Geometry: see drawing. Coordinates: mm, zero at the bounding-box minimum. A direction names the side the tool comes from. Give positions to 0.01 mm unless a question says otherwise; leave off trailing zeros. Order: outer loops, then holes, each group sorted by start corner. A loop starts at its lowest first (then second) coordinate and runs counter-clockwise, first axis right, second up. Notation, with made-up numbers: (26, 70) - (66, 70) arc R15 cw to (66, 75) - close; hole circle Ø9 at (72.25, 59). An arc over 180 degrees is marked (long way). One line per item, written item: value.
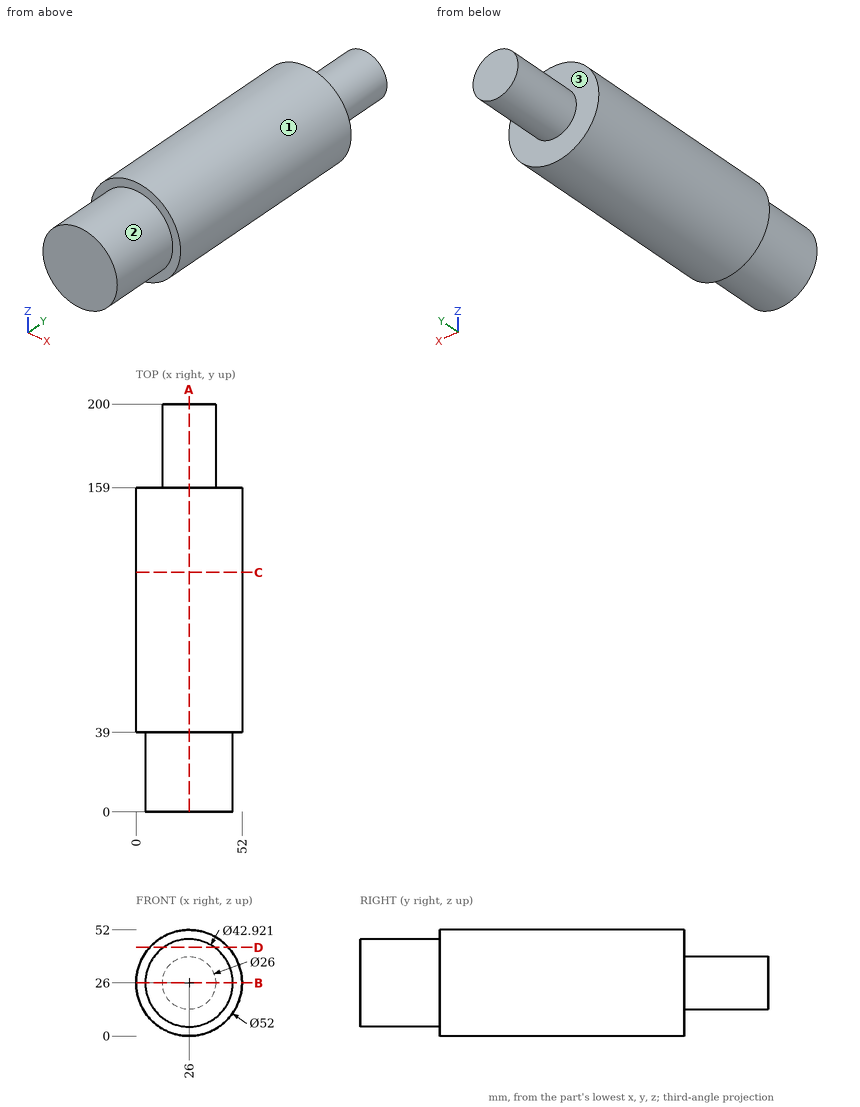
1) First-contact query: pin 1 (2 mm diameter, centred on x = 8.5, y = 156.5, fed in from -Z); pin 2 (10 mm diameter, centred on y = 35.5, z = 6, fed in from +X); pin 3 (1.5 mm diameter, centred on x = 33, z = 42, fed in from +Y); pin 4 (1.5 mm diameter, centred on x = 8, z = 46, fed in from -Y). Flat tips, straight axial feed; report the tip coordinate or a pass-through.
Answers below:
pin 1: z = 5.91
pin 2: x = 46.15
pin 3: y = 159
pin 4: through
2) Section D-D, the plane z = 43.5. Return loops of the section in (x, y), then the cut area to 3 significant figures.
Answers below:
outline: (6.77, 39) - (13.58, 39) - (13.58, 0) - (38.42, 0) - (38.42, 39) - (45.23, 39) - (45.23, 159) - (6.77, 159) - close
area: 5,580 mm^2
3) Section C-C, the plane y = 117.5. Return loops of the section in (x, z).
Answers below:
outline: circle Ø52 at (26, 26)
4) Set-up query: the marked faces 1, 2 and 3. Return all of +Z, -Z, +X, -X, +Y, -Y with unobstructed straight access to the full face (end or side cutting, diameter ignored); none if empty.
Answers below:
face 1: +Y, -Y
face 2: -Y
face 3: +Y
5) Section A-A, the plane x = 26. Return loops of the section in (y, z), then the cut area to 3 significant figures.
Answers below:
outline: (0, 4.54) - (39, 4.54) - (39, 0) - (159, 0) - (159, 13) - (200, 13) - (200, 39) - (159, 39) - (159, 52) - (39, 52) - (39, 47.46) - (0, 47.46) - close
area: 8,980 mm^2
6) Section B-B, the plane z = 26. Return loops of the section in (x, y).
Answers below:
outline: (0, 39) - (4.54, 39) - (4.54, 0) - (47.46, 0) - (47.46, 39) - (52, 39) - (52, 159) - (39, 159) - (39, 200) - (13, 200) - (13, 159) - (0, 159) - close
7) Material intervals for line 1 along Y through (x, z) = (18, 4); line 2 along Y through (x, z) = (33, 14); line 3 along X through (y, z) = (30.5, 27), sorted ascending.
Answers below:
line 1: 39 to 159
line 2: 0 to 159
line 3: 4.56 to 47.44
